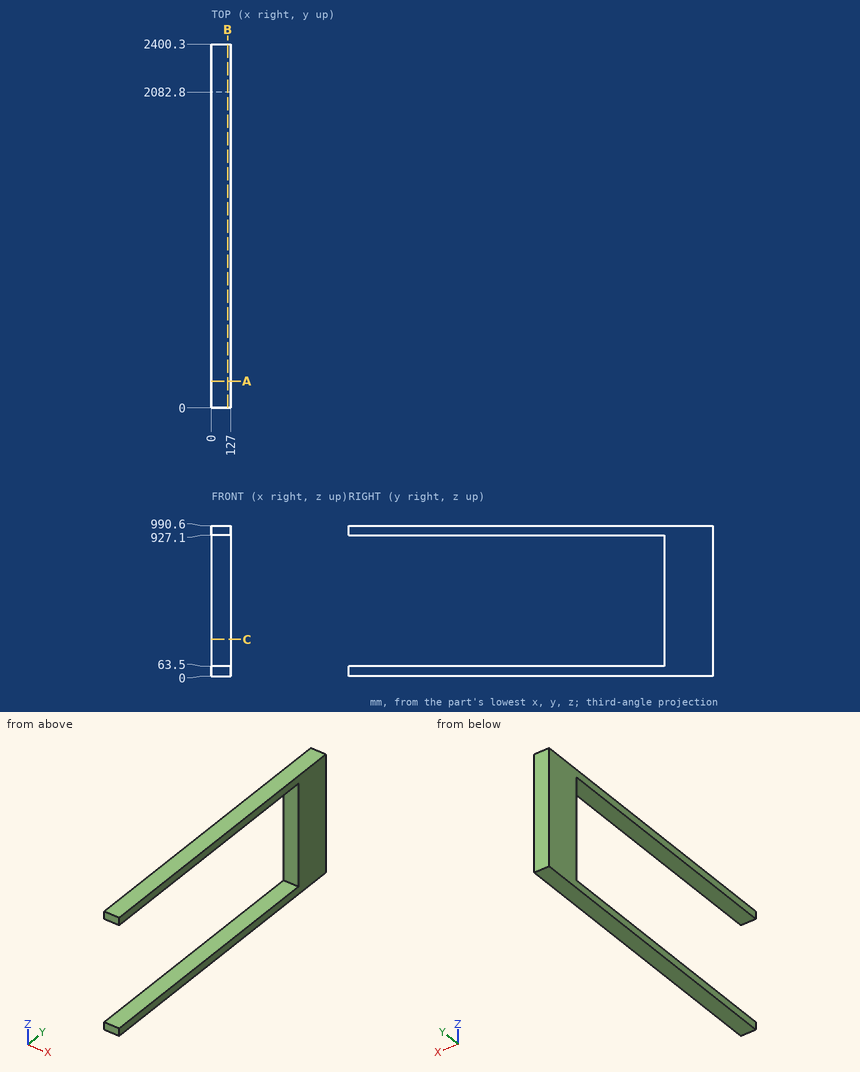
Geometry check sheet. Reference: drawing and pictorial views, mm from the part's lowest x, y, z. Coordinates: 2 decimals unless noted, no trailing zeros. Order: outer loops, then holes, each group sorted by start corner. A loop starts at its lowest first (then second) coordinate and runs counter-clockwise, first axis right, second up.
1. Sectioned sample at B-B, the plane x = 106. Record the cut outline in (y, z).
Results found:
outline: (0, 0) - (2400.3, 0) - (2400.3, 990.6) - (0, 990.6) - (0, 927.1) - (2082.8, 927.1) - (2082.8, 63.5) - (0, 63.5) - close
2. Scan lines: line 1 (Z direction, x = 118.5, y = 1194.5); line 2 (Y direction, x = 119.5, z = 782). Record each from-to range of solid material in increasing order.
Results found:
line 1: z = 0 to 63.5, 927.1 to 990.6
line 2: y = 2082.8 to 2400.3
3. Go/stop test with a flat-tipped pin: pin 1 Ø4 at (x, z) = (82, 140) entering from -Y. Record where the tip stops, or that it passes through.
Results found:
pin 1: stops at y = 2082.8
4. Sectioned sample at C-C, the plane z = 242. Record the cut outline in (x, y), and give its area (3 significant figures).
Results found:
outline: (0, 2082.8) - (127, 2082.8) - (127, 2400.3) - (0, 2400.3) - close
area: 40,300 mm2
5. Sectioned sample at A-A, the plane y = 176. Record the cut outline in (x, z).
Results found:
outline: (0, 0) - (127, 0) - (127, 63.5) - (0, 63.5) - close; (0, 927.1) - (127, 927.1) - (127, 990.6) - (0, 990.6) - close
